```python
from build123d import *

# Parameters (mm, degrees)
SKETCH1_W           = 70
SKETCH1_H           = 70
BOSS_EXTRUDE1_DEPTH = 5
SKETCH2_R           = 2.5
CUT_EXTRUDE1_DEPTH  = 5
SKETCH3_R           = 2.5
CUT_EXTRUDE2_DEPTH  = 5
SKETCH4_R           = 2.5
CUT_EXTRUDE3_DEPTH  = 5
SKETCH5_R           = 2.5
CUT_EXTRUDE4_DEPTH  = 5
SKETCH7_W           = 16
SKETCH7_H           = 16
BOSS_EXTRUDE2_DEPTH = 75
SKETCH8_W           = 8
SKETCH8_H           = 8
BOSS_EXTRUDE3_DEPTH = 25
SKETCH9_W           = 8
SKETCH9_H           = 8
BOSS_EXTRUDE4_DEPTH = 25
SKETCH10_W          = 8
SKETCH10_H          = 8
BOSS_EXTRUDE5_DEPTH = 25
SKETCH11_W          = 16
SKETCH11_H          = 4
CUT_EXTRUDE5_DEPTH  = 50
FILLET1_R           = 15
FILLET2_R           = 3


with BuildPart() as part:
    # Sketch1 → Boss-Extrude1 (new body)
    with BuildSketch(Plane(origin=(0, 0, 0), x_dir=(1, 0, 0), z_dir=(0, 1, 0))):
        Rectangle(SKETCH1_W, SKETCH1_H)
    extrude(amount=BOSS_EXTRUDE1_DEPTH)

    # Sketch2 → Cut-Extrude1 (cut)
    with BuildSketch(Plane(origin=(0, 5, 0), x_dir=(1, 0, 0), z_dir=(0, 1, 0))):
        with Locations(Location((-25, 25, 0), (0, 0, 270))):
            Circle(SKETCH2_R)
    extrude(amount=-CUT_EXTRUDE1_DEPTH, mode=Mode.SUBTRACT)

    # Sketch3 → Cut-Extrude2 (cut)
    with BuildSketch(Plane(origin=(0, 5, 0), x_dir=(1, 0, 0), z_dir=(0, 1, 0))):
        with Locations(Location((25, 25, 0), (0, 0, 270))):
            Circle(SKETCH3_R)
    extrude(amount=-CUT_EXTRUDE2_DEPTH, mode=Mode.SUBTRACT)

    # Sketch4 → Cut-Extrude3 (cut)
    with BuildSketch(Plane(origin=(0, 5, 0), x_dir=(1, 0, 0), z_dir=(0, 1, 0))):
        with Locations(Location((-25, -25, 0), (0, 0, 270))):
            Circle(SKETCH4_R)
    extrude(amount=-CUT_EXTRUDE3_DEPTH, mode=Mode.SUBTRACT)

    # Sketch5 → Cut-Extrude4 (cut)
    with BuildSketch(Plane(origin=(0, 5, 0), x_dir=(1, 0, 0), z_dir=(0, 1, 0))):
        with Locations(Location((25, -25, 0), (0, 0, 270))):
            Circle(SKETCH5_R)
    extrude(amount=-CUT_EXTRUDE4_DEPTH, mode=Mode.SUBTRACT)

    # Sketch7 → Boss-Extrude2 (add)
    with BuildSketch(Plane(origin=(0, 5, 0), x_dir=(1, 0, 0), z_dir=(0, 1, 0))):
        Rectangle(SKETCH7_W, SKETCH7_H)
    extrude(amount=BOSS_EXTRUDE2_DEPTH)

    # Sketch8 → Boss-Extrude3 (add)
    with BuildSketch(Plane.XY.offset(8)):
        with Locations((0, 47)):
            Rectangle(SKETCH8_W, SKETCH8_H)
    extrude(amount=BOSS_EXTRUDE3_DEPTH)

    # Sketch9 → Boss-Extrude4 (add)
    with BuildSketch(Plane(origin=(8, 0, 0), x_dir=(0, 0, -1), z_dir=(1, 0, 0))):
        with Locations((0, 47)):
            Rectangle(SKETCH9_W, SKETCH9_H)
    extrude(amount=BOSS_EXTRUDE4_DEPTH)

    # Sketch10 → Boss-Extrude5 (add)
    with BuildSketch(Plane.ZY.offset(8)):
        with Locations((0, 47)):
            Rectangle(SKETCH10_W, SKETCH10_H)
    extrude(amount=BOSS_EXTRUDE5_DEPTH)

    # Sketch11 → Cut-Extrude5 (cut)
    with BuildSketch(Plane(origin=(0, 80, 0), x_dir=(1, 0, 0), z_dir=(0, 1, 0))):
        with Locations((0, 6)):
            Rectangle(SKETCH11_W, SKETCH11_H)
    extrude(amount=-CUT_EXTRUDE5_DEPTH, mode=Mode.SUBTRACT)

    # Fillet1
    fillet1_edges = [part.edges().sort_by_distance(p)[0] for p in [
        (8, 5, 0),
        (0, 5, -8),
        (-8, 5, 0),
        (0, 5, 8),
    ]]
    fillet(fillet1_edges, radius=FILLET1_R)

    # Fillet2
    fillet2_edges = [part.edges().sort_by_distance(p)[0] for p in [
        (4, 47, 8),
        (0, 51, 8),
        (-4, 47, 8),
        (0, 43, 8),
        (8, 51, 0),
        (8, 47, 4),
        (8, 43, 0),
        (-8, 47, 4),
        (-8, 51, 0),
        (-8, 43, 0),
    ]]
    fillet(fillet2_edges, radius=FILLET2_R)


solid = part.part
```
CAD build for the part. Positions are in the model's coordinates, mm. A direction names the side the tool comes from. Coordinates: 2 decimals unless noted, no trailing zeros. Order: outer loops, then holes, each group sorted by start corner. A loop starts at its lowest first (then second) coordinate and runs counter-clockwise, first axis right, second up.
(1) Saw through at B-B, the plane x = -25. Write the cut outline in (y, z), and give its area (3 significant figures).
Solution:
outline: (0, -35) - (5, -35) - (5, -27.5) - (0, -27.5) - close; (0, -22.5) - (5, -22.5) - (5, 22.5) - (0, 22.5) - close; (0, 27.5) - (5, 27.5) - (5, 35) - (0, 35) - close; (43, -4) - (51, -4) - (51, 4) - (43, 4) - close
area: 364 mm2
(2) Drill centre lines: L1, parallel to X at y = 2.5, z = 25; L2, parallel to Y at x = 0, z = 28; L3, parallel to Y at x = -29, z = -8. Where is each one in solid material? Low to high.
Solution:
L1: x = -35 to -27.5, -22.5 to 22.5, 27.5 to 35
L2: y = 0 to 5, 43 to 51
L3: y = 0 to 5
(3) Saw through at D-D, the plane x = 21. Write the cut outline in (y, z).
Solution:
outline: (0, -35) - (5, -35) - (5, -23) arc R15 cw to (5.13, -21) - (5.13, 21) arc R15 cw to (5, 23) - (5, 35) - (0, 35) - close; (43, -4) - (51, -4) - (51, 4) - (43, 4) - close
(4) Saw through at A-A, the plane z = 25. Write the cut outline in (x, y), and give its area (3 significant figures).
Solution:
outline: (-35, 0) - (-27.5, 0) - (-27.5, 5) - (-35, 5) - close; (-22.5, 0) - (22.5, 0) - (22.5, 5) - (-22.5, 5) - close; (-4, 43) - (4, 43) - (4, 51) - (-4, 51) - close; (27.5, 0) - (35, 0) - (35, 5) - (27.5, 5) - close
area: 364 mm2
(5) Saw through at C-C, the plane z = -25. Write the cut outline in (x, y), and give its area (3 significant figures).
Solution:
outline: (-35, 0) - (-27.5, 0) - (-27.5, 5) - (-35, 5) - close; (-22.5, 0) - (22.5, 0) - (22.5, 5) - (-22.5, 5) - close; (27.5, 0) - (35, 0) - (35, 5) - (27.5, 5) - close
area: 300 mm2
(6) Mould opens along Y. For faces 1 (the face through (0.32, 7.62, 14.53)), 2 (the face through (0, 30, -6)), 3 (the face through (-22, 47, 4)) say: released by +Y, released by -Y, zero draft, split by the parting line, or undercut.
Solution:
face 1: undercut
face 2: released by +Y
face 3: zero draft
(7) Which spindle directions (+Z, -Z, +X, -X, +Y, -Y) get a long thin tool onto all of the face, cutting with end or side? Do faces 4 (the face through (0, 43, 22)), 5 (the face through (-22, 51, 0)), 6 (the face through (-8.52, 47.1, 5.31)). Say none if no direction does.
Solution:
face 4: +Z, +X, -X
face 5: +Z, -Z, -X, +Y
face 6: +Z, -X, +Y
(8) Pin check, flat tips, straight feed: pin 1 Ø8 at (x, y) = (-3, 55.5) entering from +Z; pin 2 Ø8 at (x, y) = (-0.5, 23) entering from -Z; pin 3 Ø12 at (x, y) = (-16.5, 41.5) entering from -Z; pin 4 Ø10 at (x, y) = (16.5, 68) entering from +Z. Stop position of each tip, or through.
Solution:
pin 1: stops at z = 9.34
pin 2: stops at z = -8.03
pin 3: stops at z = -4
pin 4: passes through
